from build123d import *

# Parameters (mm, degrees)
SKETCH1_R           = 40
BOSS_EXTRUDE1_DEPTH = 10
SKETCH2_R           = 10
BOSS_EXTRUDE2_DEPTH = 250
SKETCH3_R           = 10
BOSS_EXTRUDE3_DEPTH = 30


with BuildPart() as part:
    # Sketch1 → Boss-Extrude1 (new body)
    with BuildSketch(Plane.XY):
        Circle(SKETCH1_R)
    extrude(amount=BOSS_EXTRUDE1_DEPTH)

    # Sketch2 → Boss-Extrude2 (add)
    with BuildSketch(Plane.XY.offset(10)):
        Circle(SKETCH2_R)
    extrude(amount=BOSS_EXTRUDE2_DEPTH)

    # Sketch3 → Boss-Extrude3 (add)
    with BuildSketch(Plane(origin=(0, 0, 0), x_dir=(-1, 0, 0), z_dir=(0, 0, -1))):
        with Locations((26.998561916, 0)):
            Circle(SKETCH3_R)
    extrude(amount=BOSS_EXTRUDE3_DEPTH)


solid = part.part
The model under review builds one solid part; all positions refer to its coordinate system, in mm. A direction names the side the tool comes from. Give positions to 0.01 mm unless a question says otherwise; leave off trailing zeros. Order: outer loops, then holes, each group sorted by start corner. A loop starts at its lowest first (then second) coordinate and runs counter-clockwise, first axis right, second up. Notation, with made-up numbers: M 86.5,82 L 132.5,82 A25 cw 132.5,111 Z; hole C 69.25,87.25 d1. An arc over 180 degrees is marked long. Use one line per item in the form item = value. Start each with the question number.
Item 1: For faces 1 (the flat face through (8, -8, 10)), 2 (the flat face through (0, 0, 260)), 3 (the cylindrical face through (-36.54, 3, -14.79)), list the 3-axis set-ups (+Z, -Z, +X, -X, +Y, -Y) from which the entire face can be reached by the end or side of a thin tool; tool diameter is ignored.
Item 2: We need section B-B on y = 0. Give the boundary of the cut face in (x, z), plus the area to 3 significant figures.
Item 3: To check wall thickness, follow line 1 along Z through (x, y) = (-22, 13); line 2 along Z through (x, y) = (7, 5.5); line 3 along Y through (x, z) = (1, 124). State the ranges of each line that lie inside material, in increasing order. Write a range as from..to.
Item 4: We need section D-D on y = 24. Give the boundary of the cut face in (x, z), plus the area to 3 significant figures.
Item 5: We need section A-A on x = 0. Give the boundary of the cut face in (y, z).
Item 6: We need section C-C on z = 200.5. Give the boundary of the cut face in (x, y), plus the area to 3 significant figures.
Item 7: Insertion check: pin 1 Ø4 at (x, y) = (-2, 30.5) entering from +Z; pin 2 Ø4 at (x, y) = (24.5, -22) entering from -Z; pin 3 Ø4 at (x, z) = (4.5, 147) entering from +Y. Each pin has a flat end and moves straight along its axis. Give the tip position at first contact, or say it passes through.
Completed:
q1.face_1 = +Z
q1.face_2 = +Z, +X, -X, +Y, -Y
q1.face_3 = -Z
q2.outline = M -40,0 L -37,0 L -37,-30 L -17,-30 L -17,0 L 40,0 L 40,10 L 10,10 L 10,260 L -10,260 L -10,10 L -40,10 Z
q2.area = 6,400 mm²
q3.line_1 = 0..10
q3.line_2 = 0..260
q3.line_3 = -9.95..9.95
q4.outline = M -32,0 L 32,0 L 32,10 L -32,10 Z
q4.area = 640 mm²
q5.outline = M -40,0 L 40,0 L 40,10 L 10,10 L 10,260 L -10,260 L -10,10 L -40,10 Z
q6.outline = C 0,0 d20
q6.area = 314 mm²
q7.pin_1 = 10
q7.pin_2 = 0
q7.pin_3 = 9.68
